```python
from build123d import *

# Parameters (mm, degrees)
SKETCH1_W           = 158.75
SKETCH1_H           = 57.15
BOSS_EXTRUDE1_DEPTH = 29.591
SKETCH2_W           = 132.588
SKETCH2_H           = 32.258
CUT_EXTRUDE1_DEPTH  = 90.401054418
CUT_EXTRUDE2_DEPTH  = 14.351
FILLET1_R           = 2.38125
SKETCH8_W           = 15.24
SKETCH8_H           = 10.16
CUT_EXTRUDE5_DEPTH  = 25.781
SKETCH5_W           = 158.75
SKETCH5_H           = 57.15
BOSS_EXTRUDE2_DEPTH = 0.889
CUT_EXTRUDE3_REACH  = 91.699
SKETCH7_R           = 20
CUT_EXTRUDE4_DEPTH  = 5


with BuildPart() as part:
    # Sketch1 → Boss-Extrude1 (new body)
    with BuildSketch(Plane.XY):
        Rectangle(SKETCH1_W, SKETCH1_H)
    extrude(amount=BOSS_EXTRUDE1_DEPTH)

    # Sketch2 → Cut-Extrude1 (cut, through all)
    with BuildSketch(Plane(origin=(0, 0, 0), x_dir=(-1, 0, 0), z_dir=(0, 0, -1))):
        with Locations((2.159, 0)):
            Rectangle(SKETCH2_W, SKETCH2_H)
    extrude(amount=-CUT_EXTRUDE1_DEPTH, mode=Mode.SUBTRACT)

    # Sketch4 → Cut-Extrude2 (cut)
    with BuildSketch(Plane(origin=(0, 0, 0), x_dir=(-1, 0, 0), z_dir=(0, 0, -1))):
        Polygon((-74.803, 5.08), (-89.535, 5.08), (-89.535, 3.5), (-79.375, 3.5), (-79.375, 0), (-64.135, 0), (-64.135, 5.08), (-64.135, 16.129), (-74.803, 16.129), align=None)
    cut_extrude2 = extrude(amount=-CUT_EXTRUDE2_DEPTH, mode=Mode.SUBTRACT)

    # Mirror1: Cut-Extrude2 across plane
    add(cut_extrude2.mirror(Plane.ZX), mode=Mode.SUBTRACT)

    # Fillet1
    fillet1_edges = [part.edges().sort_by_distance(p)[0] for p in [
        (74.803, 16.129, 7.1755),
        (74.803, -16.129, 7.1755),
    ]]
    fillet(fillet1_edges, radius=FILLET1_R)

    # Sketch8 → Cut-Extrude5 (cut)
    with BuildSketch(Plane(origin=(0, 0, 0), x_dir=(-1, 0, 0), z_dir=(0, 0, -1))):
        with Locations((-71.755, 0)):
            Rectangle(SKETCH8_W, SKETCH8_H)
    extrude(amount=-CUT_EXTRUDE5_DEPTH, mode=Mode.SUBTRACT)

    # Sketch5 → Boss-Extrude2 (add)
    with BuildSketch(Plane.XY.offset(29.591)):
        Rectangle(SKETCH5_W, SKETCH5_H)
    extrude(amount=BOSS_EXTRUDE2_DEPTH)

    # Cut-Extrude3: up to this face of the body (flat: up to its plane)
    cut_extrude3_end = Plane(part.part.faces().sort_by_distance((-2.159, 0, 29.591))[0])
    # Sketch6 → Cut-Extrude3 (cut, up to the picked face)
    with BuildSketch(Plane(origin=(0, 0, 0), x_dir=(-1, 0, 0), z_dir=(0, 0, -1)), mode=Mode.PRIVATE) as cut_extrude3_sk1:
        with BuildLine():
            Line((-64.135, -16.129), (-64.135, 16.129))
            ThreePointArc((-64.135, 16.129), (-61.75375, 18.51025), (-59.3725, 16.129))
            Line((-59.3725, 16.129), (-59.3725, -16.129))
            ThreePointArc((-59.3725, -16.129), (-61.75375, -18.51025), (-64.135, -16.129))
        make_face()
    cut_extrude3_tool1 = split(extrude(cut_extrude3_sk1.sketch, amount=-CUT_EXTRUDE3_REACH, mode=Mode.PRIVATE), bisect_by=cut_extrude3_end, keep=Keep.BOTH, mode=Mode.PRIVATE)
    # Sketch6 → Cut-Extrude3 (cut, up to the picked face)
    with BuildSketch(Plane(origin=(0, 0, 0), x_dir=(-1, 0, 0), z_dir=(0, 0, -1)), mode=Mode.PRIVATE) as cut_extrude3_sk2:
        with BuildLine():
            Line((68.453, -16.129), (68.453, 16.129))
            ThreePointArc((68.453, 16.129), (66.07175, 18.51025), (63.6905, 16.129))
            Line((63.6905, 16.129), (63.6905, -16.129))
            ThreePointArc((63.6905, -16.129), (66.07175, -18.51025), (68.453, -16.129))
        make_face()
    cut_extrude3_tool2 = split(extrude(cut_extrude3_sk2.sketch, amount=-CUT_EXTRUDE3_REACH, mode=Mode.PRIVATE), bisect_by=cut_extrude3_end, keep=Keep.BOTH, mode=Mode.PRIVATE)
    add(cut_extrude3_tool1.solids().sort_by(Axis((61.75375, 0, 0), (0, 0, 1)))[0], mode=Mode.SUBTRACT)
    add(cut_extrude3_tool2.solids().sort_by(Axis((-66.07175, 0, 0), (0, 0, 1)))[0], mode=Mode.SUBTRACT)

    # Sketch7 → Cut-Extrude4 (cut)
    with BuildSketch(Plane(origin=(0, 0, 0), x_dir=(-1, 0, 0), z_dir=(0, 0, -1))):
        with Locations((31.75, 0)):
            Circle(SKETCH7_R)
    extrude(amount=-CUT_EXTRUDE4_DEPTH, mode=Mode.SUBTRACT)


solid = part.part
```
Could you check a few things on this model? Use its own coordinates, in mm. A direction names the side the tool comes from. Give positions to 0.01 mm unless a question says otherwise; leave off trailing zeros. Order: outer loops, then holes, each group sorted by start corner. A loop starts at its lowest first (then second) coordinate and runs counter-clockwise, first axis right, second up.
Q1. I'm going to push flat-ended pins straight in: P1, Ø5.5, axis at x = 68.5, y = 12.5, coming from the -Z side; P2, Ø4, axis at x = -2, y = 19.5, coming from the -Z side; P3, Ø3, axis at x = 44.5, y = -7.5, coming from the -Z side. Where does each tip first touch, or does it pass through?
Q2. For faces 5 (the flat face through (-32, 18, 5)), 6 (the flat face through (74, -5.08, 16)), 7 (the flat face through (-1, 28.575, 15)), which set-ups out of +Z, -Z, +X, -X, +Y, -Y let a thin tool reach every point of the face, with its end or its side?
Q3. Suppose I cut it at C-C, the plane x = 66. Write out the boundary of the cut face in (y, z) (3 decimals), and give its area (3 significant figures).
Q4. Suppose I cut it at A-A, the plane z = 28. Write out the boundary of the cut face in (x, y) (1 decimal), and give its area (3 significant figures).
Q5. If I drill on line 1 along X through (y, z) = (-14, 21) (3 decimals); line 2 along Y through (x, z) = (1.5, 12) (3 decimals); line 3 along X through (y, z) = (-7.5, 6) (3 decimals), over which ranges is the centre line in solid material (lowest first)?
Q6. We'd pull the mould along X, two halves only. Please class faces 1 (the flat face through (-1, 0, 30.48)), 2 (the flat face through (-68.453, 0, 15)), 3 (the flat face through (-3, 0, 29.591)), 4 (the flat face through (-79.375, 0, 15)): +X half, -X half, draft (parallel to the pull), parting line (faces both ways), or undercut.
Q7. Suppose I cut it at B-B, the plane y = -8. Write out the boundary of the cut face in (x, z) (3 decimals), and give its area (3 significant figures).
Solution:
1. P1: stops at z = 14.35
1. P2: stops at z = 0
1. P3: stops at z = 29.59
2. face 5: -Z
2. face 6: -Z, +X
2. face 7: +Z, -Z, +X, -X, +Y
3. outline: (-28.575, 0) - (-16.129, 0) - (-16.129, 14.351) - (-5.08, 14.351) - (-5.08, 25.781) - (5.08, 25.781) - (5.08, 14.351) - (16.129, 14.351) - (16.129, 0) - (28.575, 0) - (28.575, 30.48) - (-28.575, 30.48) - close
3. area: 1,160 mm2
4. outline: (-79.4, -28.6) - (79.4, -28.6) - (79.4, 28.6) - (-79.4, 28.6) - close; hole (-68.5, -16.1) arc R2.4 ccw to (-63.7, -16.1) - (59.4, -16.1) arc R2.4 ccw to (64.1, -16.1) - (64.1, 16.1) arc R2.4 ccw to (59.4, 16.1) - (-63.7, 16.1) arc R2.4 ccw to (-68.5, 16.1) - close
4. area: 4,760 mm2
5. line 1: x = -79.375 to -68.453, 64.135 to 79.375
5. line 2: y = -28.575 to -16.129, 16.129 to 28.575
5. line 3: x = -79.375 to -68.453, 74.803 to 79.375
6. face 1: draft
6. face 2: undercut
6. face 3: undercut
6. face 4: -X half
7. outline: (-79.375, 0) - (-68.453, 0) - (-68.453, 29.591) - (64.135, 29.591) - (64.135, 14.351) - (74.803, 14.351) - (74.803, 0) - (79.375, 0) - (79.375, 30.48) - (-79.375, 30.48) - close
7. area: 762 mm2
